Source: CAD feature listing. Evaluate the final solid. Frame: model axes, mm. A direction names the side the tool comes from. Give positions to 0.01 mm unless a question says otherwise; leave off trailing zeros. Order: outer loops, then holes, each group sorted by start corner. A loop starts at its lowest first (then second) coordinate and runs counter-clockwise, first axis right, second up. Notation, with made-up numbers: (14, 11) - (22, 11) arc R25 ccw to (22, 33) - close; hole circle Ø7 at (-0.75, 1). An arc over 180 degrees is marked (long way). Use CSV: the item, a comma, the result in double quotes.
Autodesk Inventor part; units mm, degrees
ref_plane "Work Plane1" through (55, 0, 0) normal (1, 0, 0) x (0, 0, -1)
ref_plane "YZ Plane" through (0, 0, 0) normal (1, 0, 0) x (0, 1, 0)
ref_plane "XZ Plane" through (0, 0, 0) normal (0, 1, 0) x (-1, 0, 0)
sketch "Sketch1" plane through (0, 0, 0) normal (0, 0, 1) x (1, 0, 0)
  line L0 (0, 0) -> (0, 350)
  line L1 (0, 350) -> (110, 350)
  line L2 (110, 350) -> (110, 0)
  line L3 (114, 0) -> (114, 354)
  line L4 (114, 354) -> (-4, 354)
  line L5 (-4, 354) -> (-4, 0)
  line L6 (-4, 0) -> (0, 0)
  line L7 (110, 0) -> (114, 0)
  dimension "d0" = 350
  dimension "d1" = 110
  dimension "d2" = 4
extrude "Extrusion1" add sketch "Sketch1" along normal blind 150
sketch "Sketch2" plane through (-4, 0, 0) normal (-1, 0, 0) x (0, 0, 1)
  line L0 (0, 354) -> (150, 354)
  line L1 (0, 0) -> (150, 0)
  line L2 (75, 0) -> (75, 100) construction
  circle A0 centre (75, 100) radius 17.5
  line L3 (60, 0) -> (60, 90.9861)
  line L4 (90, 0) -> (90, 90.9861)
  circle A1 centre (100, 100) radius 31 construction
  line L5 (75, 100) -> (53.0797, 121.9203) construction
  circle A2 centre (53.0797, 121.9203) radius 2.55
  circle A3 centre (53.0797, 78.0797) radius 2.55
  circle A4 centre (96.9203, 78.0797) radius 2.55
  circle A5 centre (96.9203, 121.9203) radius 2.55
  point P0 (60, 0)
  point P1 (90, 0)
  dimension "d5" = 100
  dimension "d6" = 15
  dimension "d7" = 15
  dimension "d12" = 35
  dimension "d13" = 62
  dimension "d23" = 5.1
  dimension "d26" = 360
extrude "Extrusion2" cut sketch "Sketch2" against normal blind 200
sketch "Sketch4" plane through (-4, 0, 0) normal (-1, 0, 0) x (0, 0, 1)
  arc A0 (90, 90.9861) -> (60, 90.9861) centre (75, 100) ccw construction
  line L0 (15, 75) -> (135, 75) construction
  line L1 (135, 75) -> (135, 125) construction
  line L2 (135, 125) -> (15, 125) construction
  line L3 (15, 125) -> (15, 75) construction
  line L4 (15, 75) -> (135, 125) construction
  line L5 (135, 75) -> (15, 125) construction
  circle A1 centre (15, 125) radius 3.05
  circle A2 centre (15, 75) radius 3.05
  circle A3 centre (135, 75) radius 3.05
  circle A4 centre (135, 125) radius 3.05
  point P0 (0, 0)
  dimension "d33" = 120
  dimension "d34" = 50
  dimension "d35" = 6.1
extrude "Extrusion4" cut sketch "Sketch4" against normal blind 5
ref_plane "Work Plane1" through (55, 0, 0) normal (1, 0, 0) x (0, 0, -1)
sketch "Sketch5" plane through (-4, 354, 0) normal (0, 1, 0) x (1, 0, 0)
  line L0 (118, 0) -> (0, 0)
  line L1 (0, 0) -> (0, -150)
  line L2 (118, -150) -> (0, -150)
  line L3 (118, 0) -> (118, -150)
  line L4 (4, -150) -> (114, -150)
  line L5 (59, -150) -> (59, 0) construction
  line L6 (4, 0) -> (114, 0)
  circle A0 centre (59, -75) radius 5
  circle A1 centre (59, -75) radius 47.5 construction
  line L7 (59, -75) -> (11.5, -75) construction
  line L8 (59, -75) -> (25.4124, -108.5876) construction
  circle A2 centre (25.4124, -108.5876) radius 3.05
  circle A3 centre (92.5876, -108.5876) radius 3.05
  circle A4 centre (92.5876, -41.4124) radius 3.05
  circle A5 centre (25.4124, -41.4124) radius 3.05
  dimension "d38" = 10
  dimension "d41" = 95
  dimension "d42" = 6.1
  dimension "d43" = 45
  dimension "d46" = 360
extrude "Extrusion5" cut sketch "Sketch5" against normal blind 20 contours A2 | A3 | A4 | A5
properties part number "CShape"
Item 1: Mould query, pull axis Y, two halves, no side actions, for faces 1 (the cylindrical face through (-2.028, 128.024, 14.603)), 2 (the flat face through (54, 350, 74)), 3 (the cylindrical face through (91.5, 352, 40.5)), 4 (the cylindrical face through (111.972, 117.492, 75.517)). Classes: released by +Y, released by -Y, zero draft, split by the parting line, or undercut.
Filled in:
face 1,"undercut"
face 2,"released by -Y"
face 3,"zero draft"
face 4,"undercut"
Item 2: Material intervals for line 1 (X direction, y = 272.5, z = 112); line 2 (Y direction, x = -1.2, z = 15); line 3 (Y direction, x = 109, z = 55.5), sorted ascending. Write a range as from..to.
Filled in:
line 1,"x = -4..0, 110..114"
line 2,"y = 0..71.95, 78.05..121.95, 128.05..354"
line 3,"y = 350..354"
Item 3: Section A-A on y = 29. Return the cut outline in (x, z), then the cut area to 3 significant figures.
Filled in:
outline,"(-4, 0) - (0, 0) - (0, 60) - (-4, 60) - close; (-4, 90) - (0, 90) - (0, 150) - (-4, 150) - close; (110, 0) - (114, 0) - (114, 60) - (110, 60) - close; (110, 90) - (114, 90) - (114, 150) - (110, 150) - close"
area,"960 mm2"
Item 4: First-contact query: pin 1 (5 mm diameter, centred on x = 66, z = 42, fed in from -Y); pin 2 (5 mm diameter, centred on y = 75, z = 15, fed in from -X); pin 3 (5.5 mm diameter, centred on x = 88.59, z = 108.59, fed in from -Y). Flat tips, straight axial feed; report the tip coordinate or a pass-through.
Filled in:
pin 1,"stops at y = 350"
pin 2,"stops at x = 110"
pin 3,"passes through"
Item 5: Set-up query: faces 5 (the flat face through (110, 177, 74)), 6 (the cylindrical face through (-2.028, 73.832, 137.817)), 7 (the cylindrical face through (91.497, 352.028, 107.671)). Return all of +Z, -Z, +X, -X, +Y, -Y with unobstructed straight access to the full face (end or side cutting, diameter ignored); none if empty.
Filled in:
face 5,"+Z, -Z, -Y"
face 6,"-X"
face 7,"+Y, -Y"
Item 6: Section C-C on y = 202. Return the cut outline in (x, z).
Filled in:
outline,"(-4, 0) - (0, 0) - (0, 150) - (-4, 150) - close; (110, 0) - (114, 0) - (114, 150) - (110, 150) - close"
Item 7: Section D-D on y = 100. Return the cut outline in (x, z).
Filled in:
outline,"(-4, 0) - (0, 0) - (0, 57.5) - (-4, 57.5) - close; (-4, 92.5) - (0, 92.5) - (0, 150) - (-4, 150) - close; (110, 0) - (114, 0) - (114, 57.5) - (110, 57.5) - close; (110, 92.5) - (114, 92.5) - (114, 150) - (110, 150) - close"
Item 8: Section B-B on z = 27.5. Return the cut outline in (x, y).
Filled in:
outline,"(-4, 0) - (0, 0) - (0, 350) - (110, 350) - (110, 0) - (114, 0) - (114, 354) - (-4, 354) - close"
